from build123d import *

# Parameters (mm, degrees)
RESSALTO_EXTRUS_O1_DEPTH = 4
ESBO_O3_R                = 3.265
CORTE_EXTRUS_O1_DEPTH    = 10
CHANFRO1_SIZE            = 4


with BuildPart() as part:
    # Esboço2 → Ressalto-extrusão1 (new body)
    with BuildSketch(Plane(origin=(0, 0, 0), x_dir=(1, 0, 0), z_dir=(0, 1, 0))):
        with BuildLine():
            Line((-4.324324324, 9), (5.675675676, 9))
            ThreePointArc((5.675675676, 9), (14.675675676, 0), (5.675675676, -9))
            Line((5.675675676, -9), (-4.324324324, -9))
            ThreePointArc((-4.324324324, -9), (-13.324324324, 0), (-4.324324324, 9))
        make_face()
    extrude(amount=RESSALTO_EXTRUS_O1_DEPTH)

    # Esboço3 → Corte-extrusão1 (cut)
    with BuildSketch(Plane(origin=(0, 0, 0), x_dir=(-1, 0, 0), z_dir=(0, -1, 0))):
        with Locations(Location((0, 0, 0), (0, 0, 90))):
            Circle(ESBO_O3_R)
    extrude(amount=-CORTE_EXTRUS_O1_DEPTH, mode=Mode.SUBTRACT)

    # Chanfro1
    chanfro1_edges = [part.edges().sort_by_distance(p)[0] for p in [
        (0, 0, 3.265),
    ]]
    chamfer(chanfro1_edges, length=CHANFRO1_SIZE - 0.0001)  # a hair under: the kernel refuses the full size


solid = part.part
Part model, mm, in its own coordinate system. Coordinates: 2 decimals unless noted, no trailing zeros. Order: outer loops, then holes, each group sorted by start corner. A loop starts at its lowest first (then second) coordinate and runs counter-clockwise, first axis right, second up. Notation, with made-up numbers: M -28,80 L 14,80 A35 ccw 14,119 Z; hole C -12.5,86 d7. An arc over 180 degrees is marked long. One line per question, with ' | ' between items.
Q1. Pin check, flat tips, straight feed: P1, Ø2, axis at y = 2.5, z = 4, coming from the +X side; P2, Ø2, axis at x = 11, y = 1, coming from the +Z side; P3, Ø4, axis at x = 0, z = 0, coming from the +Y side; P4, Ø1.5, axis at y = 1, z = -5.5, coming from the +X side. Stop position of each tip, or through.
A:
P1: stops at x = 14.16 | P2: stops at z = 7.89 | P3: passes through | P4: stops at x = 13.32
Q2. Slice it at C-C (y = 2.4). Give the cut face in (x, z), and give its area (3 significant figures).
A:
outline: M -4.32,-9 L 5.68,-9 A9 ccw 5.68,9 L -4.32,9 A9 ccw Z; hole C 0,0 d9.73 | area: 360 mm^2
Q3. Slice it at D-D (x = 11). Give the cut face in (y, z), and give its area (3 significant figures).
A:
outline: M 0,-7.26 L 4,-7.26 L 4,7.26 L 0,7.26 Z | area: 58.0 mm^2
Q4. Two-plate mould, pull along Z, no slides. Class faces 1 (the face through (7, 0, 4)), 2 (the face through (3.43, 3.806, 0.45)), 3 (the face through (-13.322, 1.972, 0.198)), 4 (the face through (1, 2, -9)): +Z half, -Z half, draft (parallel to the pull), parting line (faces both ways), or undercut.
A:
face 1: draft | face 2: undercut | face 3: parting line | face 4: -Z half
Q5. Drill centre lines: line 1 (Z direction, x = 0.5, y = 2.4); line 2 (X direction, y = 2.7, z = 8.25); line 3 (X direction, y = 3.75, z = 6). Where is each one in solid material? Low to high.
A:
line 1: z = -9 to -4.84, 4.84 to 9 | line 2: x = -7.92 to 9.27 | line 3: x = -11.03 to 12.38
